```python
from build123d import *

# Parameters (mm, degrees)
SKETCH_1_R          = 2.65
SKETCH_1_R_2        = 2.75
SKETCH_1_R_3        = 12.1
EXTRUDE_1_DEPTH     = 7
EXTRUDE_START       = -7
SKETCH_2_R          = 12.1
SKETCH_2_R_2        = 11.6
EXTRUDE_2_DEPTH     = 1.9
SKETCH_3_R          = 5.1
SKETCH_3_R_2        = 2.65
CUT_EXTRUDE_1_DEPTH = 3.5
SKETCH_4_R          = 4.25
SKETCH_4_R_2        = 2.75
EXTRUDE_3_DEPTH     = 0.5


with BuildPart() as part:
    # 草图1 → 凸台-拉伸1 (new body)
    with BuildSketch(Plane(origin=(0, 0, 0), x_dir=(1, 0, 0), z_dir=(0, 1, 0))):
        with BuildLine():
            Line((40.480150219, 0), (56.971640332, 0))
            ThreePointArc((56.971640332, 0), (61.9213878, -2.050252532), (63.971640332, -7))
            Line((63.971640332, -7), (63.971640332, -35))
            ThreePointArc((63.971640332, -35), (59.032841716, -41.689652372), (51.185512088, -38.939634494))
            Line((51.185512088, -38.939634494), (47.590395779, -33.659498976))
            ThreePointArc((47.590395779, -33.659498976), (43.546468384, -30.69695478), (38.539560652, -30.94371753))
            ThreePointArc((38.539560652, -30.94371753), (31.985820166, -32.238145), (25.43207968, -30.94371753))
            ThreePointArc((25.43207968, -30.94371753), (20.425171948, -30.69695478), (16.381244554, -33.659498976))
            Line((16.381244554, -33.659498976), (12.786128244, -38.939634494))
            ThreePointArc((12.786128244, -38.939634494), (4.938798616, -41.689652372), (0, -35))
            Line((0, -35), (0, -7))
            ThreePointArc((0, -7), (2.050252532, -2.050252532), (7, 0))
            Line((7, 0), (23.491490114, 0))
            ThreePointArc((23.491490114, 0), (31.985820166, 2.238145), (40.480150219, 0))
        make_face()
        with Locations((56.971640332, -7)):
            Circle(SKETCH_1_R, mode=Mode.SUBTRACT)
        with Locations((56.971640332, -35)):
            Circle(SKETCH_1_R_2, mode=Mode.SUBTRACT)
        with Locations((7, -23)):
            Circle(SKETCH_1_R, mode=Mode.SUBTRACT)
        with Locations((7, -7)):
            Circle(SKETCH_1_R, mode=Mode.SUBTRACT)
        with Locations((7, -35)):
            Circle(SKETCH_1_R_2, mode=Mode.SUBTRACT)
        with Locations((56.971640332, -23)):
            Circle(SKETCH_1_R, mode=Mode.SUBTRACT)
        with Locations((31.985820166, -15)):
            Circle(SKETCH_1_R_3, mode=Mode.SUBTRACT)
    extrude(amount=EXTRUDE_1_DEPTH)

    # 草图2 → 凸台-拉伸2 (add)
    with BuildSketch(Plane.XZ.offset(EXTRUDE_START)):
        with Locations((31.985820166, 15)):
            Circle(SKETCH_2_R)
        with Locations((31.985820166, 15)):
            Circle(SKETCH_2_R_2, mode=Mode.SUBTRACT)
    extrude(amount=EXTRUDE_2_DEPTH)

    # 草图3 → 切除-拉伸1 (cut)
    with BuildSketch(Plane(origin=(0, 7, 0), x_dir=(1, 0, 0), z_dir=(0, 1, 0))):
        with Locations((56.971640332, -7)):
            Circle(SKETCH_3_R)
        with Locations((56.971640332, -23)):
            Circle(SKETCH_3_R)
        with Locations((7, -23)):
            Circle(SKETCH_3_R)
        with Locations((7, -7)):
            Circle(SKETCH_3_R)
        with Locations((7, -7)):
            Circle(SKETCH_3_R_2, mode=Mode.SUBTRACT)
    extrude(amount=-CUT_EXTRUDE_1_DEPTH, mode=Mode.SUBTRACT)

    # 草图4 → 凸台-拉伸3 (add)
    with BuildSketch(Plane(origin=(0, 7, 0), x_dir=(1, 0, 0), z_dir=(0, 1, 0))):
        with Locations((7, -35)):
            Circle(SKETCH_4_R)
        with Locations((7, -35)):
            Circle(SKETCH_4_R_2, mode=Mode.SUBTRACT)
        with Locations((56.971640332, -35)):
            Circle(SKETCH_4_R)
        with Locations((56.971640332, -35)):
            Circle(SKETCH_4_R_2, mode=Mode.SUBTRACT)
    extrude(amount=EXTRUDE_3_DEPTH)

    # 草图5 → 切除-旋转1 (revolve, cut)
    with BuildSketch(Plane.XY.offset(35)):
        Polygon((12, 0), (9.65, 3.5), (7, 3.5), (7, 0), align=None)
    cut_revolve_1 = revolve(axis=Axis((7, 0, 35), (0, 1, 0)), mode=Mode.SUBTRACT)

    # 镜向1: 切除-旋转1 across plane
    add(cut_revolve_1.mirror(Plane.ZY.offset(-31.985820166)), mode=Mode.SUBTRACT)


solid = part.part
```
CAD build for the part. Positions are in the model's coordinates, mm. A direction names the side the tool comes from. Round coordinates to 2 decimals unless told otherwise and drop trailing zeros. Write each loop counter-clockwise with the first axis right and the second up, starting at its lowest first coordinate (ties: lowest second). Pieces come first, ordered by that corner, then holes. Notation, with made-up numbers: (-29.75, -17.75) - (21.25, -17.75) arc R19 ccw to (21.25, -6.75) - close; hole circle Ø1 at (2.5, -4.75). An arc over 180 degrees is marked (long way). Write item = value, one per line. Start each with the question number.
Q1. Band-saw the part on D-D (x = 49.5). Give the cut face in (y, z).
Q2. Drop flat-ended pins along their axis: pin 1 (5 mm diameter, centred on x = 7.5, z = 23.5, fed in from +Y); pin 2 (3 mm diameter, centred on x = 14.5, z = 25, fed in from +Y); pin 3 (3.5 mm diameter, centred on x = 12.5, y = 4.5, fed in from -Z). Give the stop position or say it passes through.
Q3. Band-saw the part on A-A (y = 6.25). Give the cut face in (x, z), then the cut area to 3 significant figures.
Q4. Which spindle directions (+Z, -Z, +X, -X, +Y, -Y) get a long thin tool onto all of the face, cutting with end or side? Do faces 1 (the cylindrical face through (61.025, 7.246, 33.723)), 2 (the flat face through (15, 3, 0)), 3 (the flat face through (14.61, 3.45, 36.26)). Say none if no direction does.
Q5. Probe L1, parallel to Z at x = 7, y = 6.1; L2, parallel to X at y = 1.5, z = 22; L3, parallel to X at y = 4.25, z = 25. List the from-to ranges inside material, lowest first. Write a range as from..to.
Q6. Mould opens along X. For faces 4 (the flat face through (63.972, 3, 21)), 5 (the flat face through (10, 7.5, 35)), 6 (the cylindrical face through (4.897, 1.726, 8.612)) say: pulls with the +X half, pulls with the -X half, needs draft (parallel to the pull), parting line crosses it, or undercut.
Q7. Band-saw the part on B-B (x = 33.5). Give the cut face in (y, z).
Q8. Band-saw the part on C-C (z = 23). Give the cut face in (x, y).
Answers below:
q1.outline = (0, 0) - (7, 0) - (7, 36.46) - (0, 36.46) - close
q2.pin_1 = 3.5
q2.pin_2 = 7
q2.pin_3 = 0
q3.outline = (0, 7) arc R7 ccw to (7, 0) - (23.49, 0) arc R17.24 ccw to (40.48, 0) - (56.97, 0) arc R7 ccw to (63.97, 7) - (63.97, 35) arc R7 ccw to (51.19, 38.94) - (47.59, 33.66) arc R7.5 cw to (38.54, 30.94) arc R17.24 ccw to (25.43, 30.94) arc R7.5 cw to (16.38, 33.66) - (12.79, 38.94) arc R7 ccw to (0, 35) - close; hole circle Ø10.2 at (7, 7); hole circle Ø10.2 at (7, 23); hole circle Ø5.5 at (7, 35); hole circle Ø23.2 at (31.99, 15); hole circle Ø10.2 at (56.97, 7); hole circle Ø10.2 at (56.97, 23); hole circle Ø5.5 at (56.97, 35)
q3.area = 1,490 mm2
q4.face_1 = +Y
q4.face_2 = -Z, -X, +Y, -Y
q4.face_3 = +Z, +Y, -Y
q5.L1 = 0..1.9, 12.1..17.9, 28.1..32.25, 37.75..42
q5.L2 = 0..4.55, 9.45..22.12, 41.86..54.52, 59.43..63.97
q5.L3 = 0..2.31, 11.69..25.17, 38.8..52.28, 61.66..63.97
q6.face_4 = pulls with the +X half
q6.face_5 = needs draft
q6.face_6 = undercut
q7.outline = (0, -2.17) - (7, -2.17) - (7, 3.5) - (5.1, 3.5) - (5.1, 3) - (0, 3) - close; (0, 27) - (5.1, 27) - (5.1, 26.5) - (7, 26.5) - (7, 32.17) - (0, 32.17) - close
q8.outline = (0, 0) - (4.35, 0) - (4.35, 3.5) - (1.9, 3.5) - (1.9, 7) - (0, 7) - close; (9.65, 0) - (22.91, 0) - (22.91, 5.1) - (23.59, 5.1) - (23.59, 7) - (12.1, 7) - (12.1, 3.5) - (9.65, 3.5) - close; (40.39, 5.1) - (41.06, 5.1) - (41.06, 0) - (54.32, 0) - (54.32, 3.5) - (51.87, 3.5) - (51.87, 7) - (40.39, 7) - close; (59.62, 0) - (63.97, 0) - (63.97, 7) - (62.07, 7) - (62.07, 3.5) - (59.62, 3.5) - close
